Check sheet for the modelled part. Datum: model origin and axes. Units: mm. A direction names the side the tool comes from. Coordinates: 2 decimals unless noted, no trailing zeros. Write each loop counter-clockwise with the first axis right and the second up, starting at its lowest first coordinate (ties: lowest second). Pieces come first, ordered by that corner, then holes. Notation, with made-up numbers: (13, -10.75) - (51, -10.75) arc R12 cw to (51, -2.75) - close; hole circle Ø5 at (17, 6.25). An arc over 180 degrees is marked (long way). Use one line per item in the form item = value. Start each with the question number.
1. Tool access check on faces 1 (the face through (0, -2, -29.1)), 2 (the face through (13.46, -2.46, -77.1)), 3 (the face through (28, 0, 29)). Record the directions out of +Z, -Z, +X, -X, +Y, -Y that give a thin tool (end or side, any length) a straight path to the whole face; none if there is none.
2. Cross-section at A-A on x = 36. Record the boundary of the cut face in (y, z), then the cut area to 3 significant figures.
3. Scan lines: line 1 along Z through (x, y) = (23.5, -1.15); line 2 along Z through (x, y) = (13, -2.5); line 3 along Z through (x, y) = (0, -3.1). Record each from-to range of solid material in increasing order.
4. Cross-section at B-B on z = -12.5. Record the boundary of the cut face in (x, y), then the cut area to 3 significant figures.
5. Draft check along X on faces 4 (the face through (28, -5, 29)), 5 (the face through (13, -2, 29.1)), 6 (the face through (30.42, -2.46, 116.08)). Enter one of: +X half, -X half, draft (parallel to the pull), parting line (faces both ways), or undercut.
6. Cross-section at C-C on y = -1.4. Give the number of separate pieces and of enclosed holes in the cut face, then the cut area to 3 significant figures.
7. Go/stop test with flat-tipped pins: pin 1 Ø0.8 at (x, y) = (-24, -1.5) entering from -Z (3 decimals); pin 2 Ø2.5 at (x, y) = (3, -1.5) entering from +Z; pin 3 Ø1.8 at (x, y) = (24.5, -1.5) entering from +Z. Record where each tip stops, or that it passes through.
```python
from build123d import *

# Parameters (mm, degrees)
EXTRUDE_1_DEPTH          = 5
CUT_EXTRUDE_1_DEPTH      = 170.779268463
CUT_EXTRUDE_1_DEPTH_BACK = 170.779268463
HOLE_WIZARD_M5_1_D       = 4.2


with BuildPart() as part:
    # Sketch 1 → Extrude 1 (new body)
    with BuildSketch(Plane(origin=(0, 0, 0), x_dir=(1, 0, 0), z_dir=(0, 1, 0))):
        with BuildLine():
            Line((-18.994949366, 44.644660941), (46.840858459, 110.480468766))
            ThreePointArc((46.840858459, 110.480468766), (26.307654113, -117.080772696), (-89.60126665, 79.822384171))
            ThreePointArc((-89.60126665, 79.822384171), (-83.752223837, 81.026793285), (-80.9211148, 75.768777998))
            ThreePointArc((-80.9211148, 75.768777998), (-61.199118411, 37.840868245), (-18.994949366, 44.644660941))
        make_face()
        Polygon((-11.923881554, 37.573593129), (44.644660941, 94.142135624), (41.109127035, 97.67766953), (-15.45941546, 41.109127035), align=None, mode=Mode.SUBTRACT)
        with BuildLine():
            Line((-19.89891353, 23.499999452), (-19.898913286, 25.100000259))
            ThreePointArc((-19.898913286, 25.100000259), (-18.727340196, 27.92842699), (-15.898913286, 29.09999965))
            Line((-15.898913286, 29.09999965), (15.898913286, 29.09999965))
            ThreePointArc((15.898913286, 29.09999965), (18.727340196, 27.92842699), (19.898913286, 25.100000259))
            Line((19.898913286, 25.100000259), (19.89891353, 23.499999452))
            ThreePointArc((19.89891353, 23.499999452), (20.953647337, 20.953647337), (23.499999452, 19.89891353))
            Line((23.499999452, 19.89891353), (25.100000259, 19.898913286))
            ThreePointArc((25.100000259, 19.898913286), (27.92842699, 18.727340196), (29.09999965, 15.898913286))
            Line((29.09999965, 15.898913286), (29.09999965, -15.898913286))
            ThreePointArc((29.09999965, -15.898913286), (27.92842699, -18.727340196), (25.100000259, -19.898913286))
            Line((25.100000259, -19.898913286), (23.499999452, -19.89891353))
            ThreePointArc((23.499999452, -19.89891353), (20.953647337, -20.953647337), (19.89891353, -23.499999452))
            Line((19.89891353, -23.499999452), (19.898913286, -25.100000259))
            ThreePointArc((19.898913286, -25.100000259), (18.727340196, -27.92842699), (15.898913286, -29.09999965))
            Line((15.898913286, -29.09999965), (-15.898913286, -29.09999965))
            ThreePointArc((-15.898913286, -29.09999965), (-18.727340196, -27.92842699), (-19.898913286, -25.100000259))
            Line((-19.898913286, -25.100000259), (-19.89891353, -23.499999452))
            ThreePointArc((-19.89891353, -23.499999452), (-20.953647337, -20.953647337), (-23.499999452, -19.89891353))
            Line((-23.499999452, -19.89891353), (-25.100000259, -19.898913286))
            ThreePointArc((-25.100000259, -19.898913286), (-27.92842699, -18.727340196), (-29.09999965, -15.898913286))
            Line((-29.09999965, -15.898913286), (-29.09999965, 15.898913286))
            ThreePointArc((-29.09999965, 15.898913286), (-27.92842699, 18.727340196), (-25.100000259, 19.898913286))
            Line((-25.100000259, 19.898913286), (-23.499999452, 19.89891353))
            ThreePointArc((-23.499999452, 19.89891353), (-20.953647337, 20.953647337), (-19.89891353, 23.499999452))
        make_face(mode=Mode.SUBTRACT)
        Polygon((-44.644660941, -94.142135624), (-41.109127035, -97.67766953), (15.45941546, -41.109127035), (11.923881554, -37.573593129), align=None, mode=Mode.SUBTRACT)
    extrude(amount=-EXTRUDE_1_DEPTH)

    # Sketch 5 → Cut-Extrude 1 (cut, two sides: drawn at the far end of the back side and taken through both)
    with BuildSketch(Plane(origin=(0, 0, 0), x_dir=(1, 0, 0), z_dir=(0, 1, 0)).offset(-CUT_EXTRUDE_1_DEPTH_BACK)):
        with BuildLine():
            Line((-5, -24.09999965), (5, -24.09999965))
            ThreePointArc((5, -24.09999965), (10, -29.09999965), (5, -34.09999965))
            Line((5, -34.09999965), (-5, -34.09999965))
            ThreePointArc((-5, -34.09999965), (-10, -29.09999965), (-5, -24.09999965))
        make_face()
    extrude(amount=CUT_EXTRUDE_1_DEPTH + CUT_EXTRUDE_1_DEPTH_BACK, mode=Mode.SUBTRACT)

    # Hole Wizard M5 _1 (through all)
    with Locations(Plane(origin=(0, 0, 0), x_dir=(1, 0, 0), z_dir=(0, 1, 0))):
        with Locations((23.5, 23.5), (23.5, -23.5), (-23.5, -23.5), (-23.5, 23.5)):
            Hole(HOLE_WIZARD_M5_1_D / 2)


solid = part.part
```
Final values:
q1.face_1 = +Y, -Y
q1.face_2 = -Z, +Y, -Y
q1.face_3 = +Z, -Z, +X, -X, +Y
q2.outline = (-5, -99.64) - (0, -99.64) - (0, -92.57) - (-5, -92.57) - close; (-5, -85.5) - (0, -85.5) - (0, 114.47) - (-5, 114.47) - close
q2.area = 1,040 mm²
q3.line_1 = -87.14 to -80.07, -73 to -25.6, -21.4 to -19.9, 19.9 to 21.4, 25.6 to 117.68
q3.line_2 = -76.64 to -69.57, -62.5 to -29.1, 29.1 to 38.65, 43.57 to 119.29
q3.line_3 = -63.64 to -56.57, -49.5 to -29.1, 34.1 to 49.5, 56.57 to 120
q4.outline = (-119.35, -5) - (-29.1, -5) - (-29.1, 0) - (-119.35, 0) - close; (29.1, -5) - (119.35, -5) - (119.35, 0) - (29.1, 0) - close
q4.area = 902 mm²
q5.face_4 = draft
q5.face_5 = undercut
q5.face_6 = parting line
q6.separate_pieces = 1
q6.enclosed_holes = 7
q6.area = 34,400 mm²
q7.pin_1 = -40.745
q7.pin_2 = 119.99
q7.pin_3 = 117.66
